from build123d import *

# Parameters (mm, degrees)
ESQUISSE2_R         = 3
BOSS_EXTRU_1_DEPTH  = 10
BOARD_HOLES_D       = 2
BOARD_HOLES_DEPTH   = 10
STEPPER_HOLES_D     = 2
STEPPER_HOLES_DEPTH = 10
FEET_HOLES_D        = 6
FEET_HOLES_DEPTH    = 10
CHANFREIN1_SIZE     = 1
STEPPER_DEPTH       = 1
PUMPS_DEPTH         = 5
WIRES_2_DEPTH       = 11
WEIGHT_DEPTH        = 1
WEIGHT_HOLES_D      = 3
WEIGHT_HOLES_DEPTH  = 9
ESQUISSE17_W        = 10
ESQUISSE17_H        = 10
WIRES_STEPPER_DEPTH = 10
CONG_1_R            = 3


with BuildPart() as part:
    # Esquisse2 → Boss.-Extru.1 (new body)
    with BuildSketch(Plane(origin=(0, 0, 0), x_dir=(1, 0, 0), z_dir=(0, 1, 0))):
        with BuildLine():
            Line((59.233727564, -68.232233047), (65.180063204, -74.178568687))
            ThreePointArc((65.180063204, -74.178568687), (66.418060903, -76.226353952), (66.562716933, -78.614896904))
            ThreePointArc((66.562716933, -78.614896904), (85.780525757, -95.637874651), (91.923881554, -70.710678119))
            Line((91.923881554, -70.710678119), (82.928932188, -61.715728753))
            ThreePointArc((82.928932188, -61.715728753), (80.761204675, -58.471495264), (80, -54.644660941))
            Line((80, -54.644660941), (80, 57.5))
            ThreePointArc((80, 57.5), (77.071067812, 64.571067812), (70, 67.5))
            Line((70, 67.5), (-50, 67.5))
            ThreePointArc((-50, 67.5), (-57.071067812, 64.571067812), (-60, 57.5))
            Line((-60, 57.5), (-60, -57.5))
            ThreePointArc((-60, -57.5), (-57.071067812, -64.571067812), (-50, -67.5))
            Line((-50, -67.5), (57.465960611, -67.5))
            ThreePointArc((57.465960611, -67.5), (58.422669192, -67.690301169), (59.233727564, -68.232233047))
        make_face()
        with Locations((-52.5, 40)):
            Circle(ESQUISSE2_R, mode=Mode.SUBTRACT)
        with Locations((-52.5, -40)):
            Circle(ESQUISSE2_R, mode=Mode.SUBTRACT)
    extrude(amount=BOSS_EXTRU_1_DEPTH)

    # board holes
    with Locations(Plane(origin=(0, 10, 0), x_dir=(1, 0, 0), z_dir=(0, 1, 0))):
        with Locations((-36.6, 47.1), (36.6, 47.1), (36.6, -47.1), (-36.6, -47.1)):
            Hole(BOARD_HOLES_D / 2, depth=BOARD_HOLES_DEPTH)

    # stepper holes
    with Locations(Plane(origin=(0, 10, 0), x_dir=(1, 0, 0), z_dir=(0, 1, 0))):
        with Locations((-16.8, 16.8), (16.8, 16.8), (16.8, -16.8), (-16.8, -16.8)):
            Hole(STEPPER_HOLES_D / 2, depth=STEPPER_HOLES_DEPTH)

    # feet holes
    with Locations(Plane(origin=(0, 10, 0), x_dir=(1, 0, 0), z_dir=(0, 1, 0))):
        with Locations((70, 57.5), (-50, 57.5), (-50, -57.5), (78.254846073, -72.973824527), (61.661200826, -57.5)):
            Hole(FEET_HOLES_D / 2, depth=FEET_HOLES_DEPTH)

    # Chanfrein1
    chanfrein1_edges = [part.edges().sort_by_distance(p)[0] for p in [
        (-35.6, 10, 47.1),
        (37.6, 10, 47.1),
        (37.6, 10, -47.1),
        (-35.6, 10, -47.1),
    ]]
    chamfer(chanfrein1_edges, length=CHANFREIN1_SIZE)

    # Esquisse10 → stepper (cut)
    with BuildSketch(Plane(origin=(0, 10, -10), x_dir=(1, 0, 0), z_dir=(0, -1, 0))):
        Polygon((-16.9, 31), (16.9, 31), (21, 26.9), (21, 15), (56, 15), (56, 5), (21, 5), (21, -6.9), (16.9, -11), (-16.9, -11), (-21, -6.9), (-21, 26.9), align=None)
    extrude(amount=STEPPER_DEPTH, mode=Mode.SUBTRACT)

    # Esquisse11 → pumps (cut)
    with BuildSketch(Plane(origin=(0, 10, 0), x_dir=(1, 0, 0), z_dir=(0, 1, 0))):
        with BuildLine():
            Line((-41, -67.5), (-19, -67.5))
            Line((-19, -67.5), (-19, -26.5))
            ThreePointArc((-19, -26.5), (-20.171572875, -23.671572875), (-23, -22.5))
            Line((-23, -22.5), (-37, -22.5))
            ThreePointArc((-37, -22.5), (-39.828427125, -23.671572875), (-41, -26.5))
            Line((-41, -26.5), (-41, -67.5))
        make_face()
        with BuildLine():
            Line((19, -67.5), (19, -26.5))
            ThreePointArc((19, -26.5), (20.171572875, -23.671572875), (23, -22.5))
            Line((23, -22.5), (37, -22.5))
            ThreePointArc((37, -22.5), (39.828427125, -23.671572875), (41, -26.5))
            Line((41, -26.5), (41, -67.5))
            Line((41, -67.5), (19, -67.5))
        make_face()
        with BuildLine():
            Line((41, 67.5), (19, 67.5))
            Line((19, 67.5), (19, 26.5))
            ThreePointArc((19, 26.5), (20.171572875, 23.671572875), (23, 22.5))
            Line((23, 22.5), (37, 22.5))
            ThreePointArc((37, 22.5), (39.828427125, 23.671572875), (41, 26.5))
            Line((41, 26.5), (41, 67.5))
        make_face()
        with BuildLine():
            Line((-19, 67.5), (-19, 26.5))
            ThreePointArc((-19, 26.5), (-20.171572875, 23.671572875), (-23, 22.5))
            Line((-23, 22.5), (-37, 22.5))
            ThreePointArc((-37, 22.5), (-39.828427125, 23.671572875), (-41, 26.5))
            Line((-41, 26.5), (-41, 67.5))
            Line((-41, 67.5), (-19, 67.5))
        make_face()
    extrude(amount=-PUMPS_DEPTH, mode=Mode.SUBTRACT)

    # Esquisse13 → wires 2 (cut, through all)
    with BuildSketch(Plane(origin=(0, 10, 0), x_dir=(1, 0, 0), z_dir=(0, 1, 0))):
        with BuildLine():
            Line((11, 62), (-11, 62))
            ThreePointArc((-11, 62), (-13.828427125, 60.828427125), (-15, 58))
            Line((-15, 58), (-15, 54))
            ThreePointArc((-15, 54), (-13.828427125, 51.171572875), (-11, 50))
            Line((-11, 50), (11, 50))
            ThreePointArc((11, 50), (13.828427125, 51.171572875), (15, 54))
            Line((15, 54), (15, 58))
            ThreePointArc((15, 58), (13.828427125, 60.828427125), (11, 62))
        make_face()
        with BuildLine():
            Line((-15, -58), (-15, -54))
            ThreePointArc((-15, -54), (-13.828427125, -51.171572875), (-11, -50))
            Line((-11, -50), (11, -50))
            ThreePointArc((11, -50), (13.828427125, -51.171572875), (15, -54))
            Line((15, -54), (15, -58))
            ThreePointArc((15, -58), (13.828427125, -60.828427125), (11, -62))
            Line((11, -62), (-11, -62))
            ThreePointArc((-11, -62), (-13.828427125, -60.828427125), (-15, -58))
        make_face()
    extrude(amount=-WIRES_2_DEPTH, mode=Mode.SUBTRACT)

    # Esquisse14 → weight (cut)
    with BuildSketch(Plane(origin=(0, 10, 0), x_dir=(1, 0, 0), z_dir=(0, 1, 0))):
        with BuildLine():
            Line((66.257054798, -53.581738396), (91.854434355, -77.451680998))
            ThreePointArc((91.854434355, -77.451680998), (92.150566404, -85.931793368), (83.670454034, -86.227925417))
            Line((83.670454034, -86.227925417), (58.073074477, -62.357982815))
            ThreePointArc((58.073074477, -62.357982815), (57.776942428, -53.877870445), (66.257054798, -53.581738396))
        make_face()
    extrude(amount=-WEIGHT_DEPTH, mode=Mode.SUBTRACT)

    # Weight holes
    with Locations(Plane(origin=(0, 9, 0), x_dir=(1, 0, 0), z_dir=(0, 1, 0))):
        with Locations((83.691023277, -78.04314178), (72.720717752, -67.813166379), (77.572847713, -73.705178228)):
            Hole(WEIGHT_HOLES_D / 2, depth=WEIGHT_HOLES_DEPTH)

    # Esquisse17 → wires stepper (cut, through all)
    with BuildSketch(Plane(origin=(0, 9, 0), x_dir=(1, 0, 0), z_dir=(0, 1, 0))):
        with Locations((51, 0)):
            Rectangle(ESQUISSE17_W, ESQUISSE17_H)
    extrude(amount=-WIRES_STEPPER_DEPTH, mode=Mode.SUBTRACT)

    # Congé1
    cong_1_edges = [part.edges().sort_by_distance(p)[0] for p in [
        (56, 5, -5),
        (56, 5, 5),
        (46, 4.5, 5),
        (46, 4.5, -5),
    ]]
    fillet(cong_1_edges, radius=CONG_1_R)


solid = part.part
Geometry: final body of the model. Coordinates: model frame, mm. A direction names the side the tool comes from. Give positions to 0.01 mm unless a question says otherwise; leave off trailing zeros. Order: outer loops, then holes, each group sorted by start corner. A loop starts at its lowest first (then second) coordinate and runs counter-clockwise, first axis right, second up. Notation, with made-up numbers: (43.25, -33.75) -> (64.25, -33.75) arc R22 ccw to (64.25, -15.75) -> close; hole circle Ø5 at (-20.5, 77). An arc over 180 degrees is marked (long way). Answer as a JSON object with one key per item and string values.
Q1. Draft query along Z for faces 1 (the flat face through (30, 5, 45)), 2 (the cylindrical face through (92.239, 9.507, 85.834)), 3 (the flat face through (30, 8, -22.5)). Return one class per face: released by +Z, released by -Z, zero draft, split by the parting line, or undercut.
Entries:
{"face 1": "zero draft", "face 2": "undercut", "face 3": "released by -Z"}
Q2. Section C-C (y = 6.5). State how many separate pieces and enclosed holes the cut face has, plus the area to 3 significant figures.
Entries:
{"separate pieces": "1", "enclosed holes": "16", "area": "14,700 mm^2"}
Q3. Access query for faces 4 (the flat face through (-19, 8, -47)), 5 (the flat face through (-19, 8, 47)), 6 (the cylindrical face through (-13.859, 5.07, 51.203)). Directions: +Z, -Z, +X, -X, +Y, -Y. A direction counts if a zero-diameter tool reaches every point of the face in a straight line with its end or side. Return the directions, or none.
Entries:
{"face 4": "-Z, +Y", "face 5": "+Z, +Y", "face 6": "+Y, -Y"}
Q4. First-contact query: pin 1 (17.5 mm diameter, centred on x = -29.5, z = -53.5, fed in from +Y); pin 2 (4 mm diameter, centred on y = 7, z = -41.5, fed in from +X); pin 3 (1 mm diameter, centred on y = 6, z = 62, fed in from -X); pin 4 (2.5 mm diameter, centred on x = 83.69, z = 78.04, fed in from -Y). Flat tips, straight axial feed; report the tip coordinate or a pass-through.
Entries:
{"pin 1": "stops at y = 5", "pin 2": "stops at x = 80", "pin 3": "stops at x = -59.17", "pin 4": "passes through"}
Q5. Section A-A (z = -40). Output: boundary loops of the cut face in (x, y).
Entries:
{"outline": "(-60, 0) -> (-55.5, 0) -> (-55.5, 10) -> (-60, 10) -> close; (-49.5, 0) -> (80, 0) -> (80, 10) -> (41, 10) -> (41, 5) -> (19, 5) -> (19, 10) -> (-19, 10) -> (-19, 5) -> (-41, 5) -> (-41, 10) -> (-49.5, 10) -> close"}
Q6. Section B-B (z = 31). Output: boundary loops of the cut face in (x, y).
Entries:
{"outline": "(-60, 0) -> (80, 0) -> (80, 10) -> (41, 10) -> (41, 5) -> (19, 5) -> (19, 10) -> (-19, 10) -> (-19, 5) -> (-41, 5) -> (-41, 10) -> (-60, 10) -> close"}
Q7. Material intervals for probe 1 along X at (y, z) = (7.75, -34.5); probe 2 along X at (y, z) = (3.15, 47.1); probe 3 along Z at (x, y) = (-16.8, 5.25), sorted ascending.
Entries:
{"probe 1": "x = -60 to -41, -19 to 19, 41 to 80", "probe 2": "x = -60 to -37.6, -35.6 to 35.6, 37.6 to 80", "probe 3": "z = -67.5 to -17.8, -15.8 to 15.8, 17.8 to 67.5"}
